```python
from build123d import *

# Parameters (mm, degrees)
SKETCH1_R           = 100
BOSS_EXTRUDE1_DEPTH = 50
FILLET1_R           = 10
CUT_EXTRUDE1_DEPTH  = 51
CIRPATTERN1_COUNT   = 5


with BuildPart() as part:
    # Sketch1 → Boss-Extrude1 (new body)
    with BuildSketch(Plane.XY):
        Circle(SKETCH1_R)
    extrude(amount=BOSS_EXTRUDE1_DEPTH)

    # Fillet1
    fillet1_edges = [part.edges().sort_by_distance(p)[0] for p in [
        (-100, 0, 0),
        (-100, 0, 50),
    ]]
    fillet(fillet1_edges, radius=FILLET1_R)

    # Sketch2 → Cut-Extrude1 (cut, through all)
    with BuildSketch(Plane.XY.offset(50)):
        with BuildLine():
            ThreePointArc((50.802293201, 74.290827196), (14.437611959, 54.039323714), (0, 15))
            ThreePointArc((0, 15), (36.99293279, 42.556106586), (82.610843349, 35.713422703))
            ThreePointArc((82.610843349, 35.713422703), (69.439328089, 57.255390267), (50.802293201, 74.290827196))
        make_face()
    cut_extrude1 = extrude(amount=-CUT_EXTRUDE1_DEPTH, mode=Mode.SUBTRACT)

    # CirPattern1: Cut-Extrude1 ×5 about axis
    cirpattern1_axis = Axis((0, 0, 0), (0, 0, 1))
    for i in range(1, CIRPATTERN1_COUNT):
        add(cut_extrude1.rotate(cirpattern1_axis, i * 360 / CIRPATTERN1_COUNT), mode=Mode.SUBTRACT)

    # Sketch3 → Cut-Revolve1 (revolve, cut)
    with BuildSketch(Plane(origin=(0, 0, 0), x_dir=(1, 0, 0), z_dir=(0, 1, 0))):
        with BuildLine():
            Line((0, 0), (-90, 0))
            ThreePointArc((-90, 0), (-45.620718977, -11.224313863), (0, -15))
            Line((0, -15), (0, 0))
        make_face()
        with BuildLine():
            Line((0, -50), (-90, -50))
            ThreePointArc((-90, -50), (-45.620718977, -38.775686137), (0, -35))
            Line((0, -35), (0, -50))
        make_face()
    revolve(axis=Axis((0, 0, 50), (0, 0, -1)), mode=Mode.SUBTRACT)


solid = part.part
```
Design review of the part built by this model. Coordinates are the model's own, in mm. Round coordinates to 2 decimals unless told otherwise and drop trailing zeros. Write each loop counter-clockwise with the first axis right and the second up, starting at its lowest first coordinate (ties: lowest second). Pieces come first, ordered by that corner, then holes. Notation, with made-up numbers: (-2, -18) -> (6, -18) arc R19 cw to (6, -13) -> close; hole circle Ø10 at (-14, -4). An arc over 180 degrees is marked (long way). Write item = value, one per line. Start each with the question number.
1) Clearance check with flat-ended pins moving along their axes: pin 1 (5 mm diameter, centred on x = -56, z = 29.5, fed in from -Y); pin 2 (8 mm diameter, centred on x = 25.5, y = -68, fed in from -Z); pin 3 (12 mm diameter, centred on y = 12, z = 17.5, fed in from +X). State where each tip first meets the part, or that it passes through.
2) Take a section at A-A, the plane y = 0. State the section outline as (x, z) points.
3) Take a section at B-B, the plane z = 19. State the section outline as (x, y) points, plus the area to 3 significant figures.
4) Mouldability with a two-part tool opening along X and no side actions: class faces 1 (the face through (95.38, 30.04, 24.79)), 2 (the face through (-32.665, 83.863, 25.35)) as +X half, -X half, draft (parallel to the pull), parting line (faces both ways), or undercut.
5) Wall thickness on probe 1 along X at (y, z) = (-40, 28); probe 2 along Y at (x, z) = (68.5, 8.5); probe 3 along X at (y, z) = (-23, 31): over which ranges is each line inside the solid? List them lowest first. Write a range as from..to.
6) Take a section at C-C, the plane x = 79. Count the separate pieces of the cut face and the enclosed holes in it, plus the area to 3 significant figures.
Results list:
q1.pin_1 = -84.49
q1.pin_2 = 4.21
q1.pin_3 = 99.82
q2.outline = (-100, 10) arc R10 ccw to (-90, 0) -> (-90, 50) arc R10 ccw to (-100, 40) -> close; (-74.41, 4.84) arc R277.5 cw to (27.43, 13.64) -> (27.43, 36.36) arc R277.5 cw to (-74.41, 45.16) -> close; (61.98, 7.99) arc R277.5 cw to (90, 0) arc R10 ccw to (100, 10) -> (100, 40) arc R10 ccw to (90, 50) arc R277.5 cw to (61.98, 42.01) -> close
q3.outline = circle Ø200 at (0, 0); hole (-87.83, 19.66) arc R90 ccw to (-84.77, -30.24) arc R60 ccw to (-8.82, -12.14) arc R60 cw to start; hole (-54.96, 71.27) arc R60 ccw to (-14.27, 4.64) arc R60 cw to (-8.44, 89.6) arc R90 ccw to start; hole (-45.84, -77.45) arc R90 ccw to (2.57, -89.96) arc R60 ccw to (8.82, -12.14) arc R60 cw to start; hole (0, 15) arc R60 cw to (82.61, 35.71) arc R90 ccw to (50.8, 74.29) arc R60 ccw to start; hole (14.27, 4.64) arc R60 cw to (59.49, -67.53) arc R90 ccw to (86.35, -25.36) arc R60 ccw to start
q3.area = 22,600 mm²
q4.face_1 = parting line
q4.face_2 = undercut
q5.probe_1 = -91.65..4.76, 19.82..59.43, 80.62..91.65
q5.probe_2 = -72.7..-58.38, -4.2..41.92, 58.38..72.7
q5.probe_3 = -97.32..-87.01, -18.99..8.83, 15.09..52.5, 85.09..97.32
q6.separate_pieces = 3
q6.enclosed_holes = 0
q6.area = 3,970 mm²
